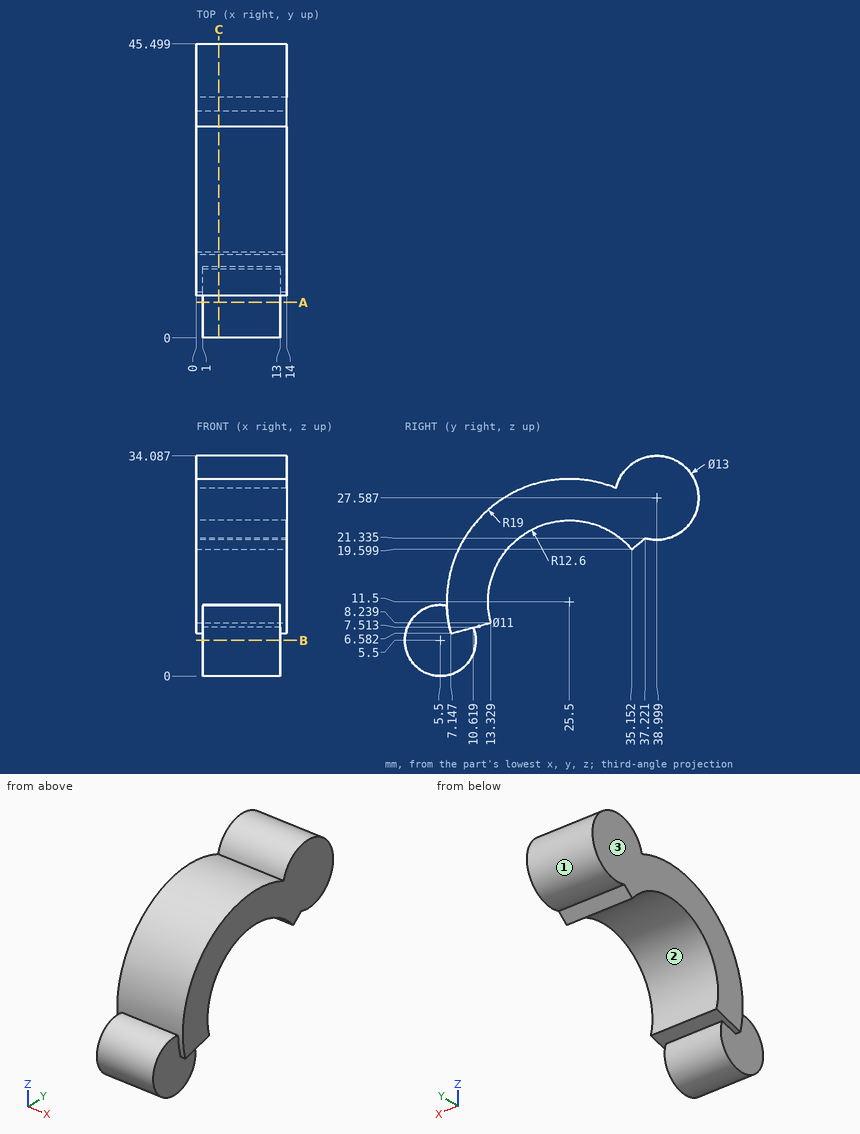
Source: three-view drawing plus pictorial views. Frame: mm from the lowest corner of the part. Round coordinates to 2 decimals unless told otherwise and drop trailing zeros. Order: outer loops, then holes, each group sorted by start corner. A loop starts at its lowest first (then second) coordinate and runs counter-clockwise, first axis right, second up. Notation, with made-up numbers: (-36, 74.5) -> (-14, 74.5) arc R29 cw to (-14, 104.5) -> close; hole circle Ø4 at (18.5, 35). An arc over 180 degrees is marked (long way). Use one line per item in the form item = value. Start each with the question number.
1. Line query: probe 1 along Y at (x, z) = (8.75, 22) (1 decimal); probe 2 along Y at (x, z) = (12.25, 12); probe 3 along Y at (x, z) = (2.25, 5.5). Output: solid intervals per line, ascending.
2. Pin query (flat end, axial travel): pin 1 Ø3 at (x, z) = (6.5, 15.5) entering from -Y (1 decimal); pin 2 Ø1.5 at (x, y) = (7.5, 11) entering from -Z (1 decimal); pin 3 Ø2 at (x, y) = (1.5, 11) entering from +Z. Return the tip coordinate at first contact, or that it passes through.
3. Cut plane C-C (x = 3.5). Return the cut outline in (y, z) (1 decimal).
4. Cut plane A-A (y = 5.5). Return the cut outline in (x, z), then the cut area to 3 significant figures.
5. Draft query along Z for the marked faces 1, 2 and 3. Return one class per face: pulls with the +Z half, pulls with the -Z half, needs draft (parallel to the pull), parting line crosses it, or undercut.
Solution:
q1.probe_1 = 9.7 to 18.5, 32.5 to 42.3
q1.probe_2 = 6.51 to 12.91
q1.probe_3 = 0 to 11
q2.pin_1 = 6.7
q2.pin_2 = 2.7
q2.pin_3 = 24.87
q3.outline = (6.5, 10.9) arc R5.5 ccw (long way) to (10.6, 7.5) -> (13.3, 8.2) arc R12.6 cw to (35.2, 19.6) -> (37.2, 21.3) arc R6.5 ccw (long way) to (32.7, 29.1) arc R19 ccw to start
q4.outline = (1, 0) -> (13, 0) -> (13, 11) -> (1, 11) -> close
q4.area = 132 mm^2
q5.face_1 = parting line crosses it
q5.face_2 = undercut
q5.face_3 = needs draft
